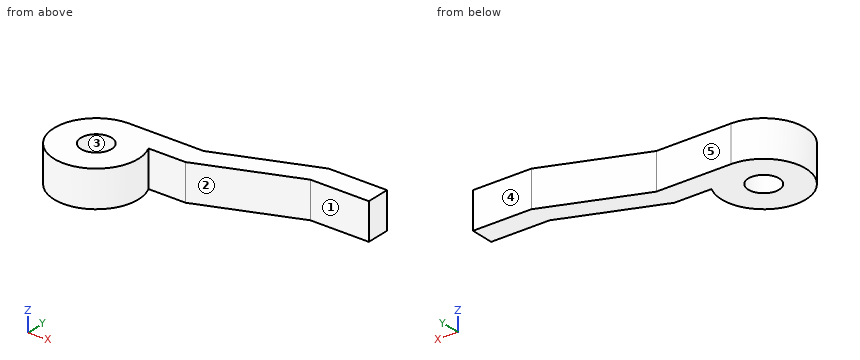
Autodesk Fusion 360 part; units mm, degrees
sketch "Sketch1" plane through (0, 0, 0) normal (0, 0, 1) x (1, 0, 0)
  circle A0 centre (0, 0) radius 0.8344
  line L0 (0, 0) -> (-2.286, 0) construction
  line L1 (0, 2.286) -> (4.064, 2.286)
  line L2 (2.0478, 1.016) -> (4.064, 1.016)
  line L3 (12.446, 4.318) -> (9.271, 4.318)
  line L4 (12.446, 4.318) -> (12.446, 3.048)
  line L5 (12.446, 3.048) -> (9.271, 3.048)
  line L6 (4.064, 2.286) -> (9.271, 4.318)
  line L7 (4.064, 1.016) -> (9.271, 3.048)
  arc A1 (0, 2.286) -> (2.0478, 1.016) centre (0, 0) ccw
  dimension "d1" = 1.6688
  dimension "d2" = 4.572
  dimension "d9" = 3.175
  dimension "d10" = 1.27
  dimension "d11" = 3.175
extrude "Extrude1" add sketch "Sketch1" along normal blind 1.9812
The model under review builds one solid part; all positions refer to its coordinate system, in mm. Face numbers are marked on the shaded views. A direction names the side the tool comes from. Round coordinates to 2 decimals unless told otherwise and drop trailing zeros. Loops run counter-clockwise (first coordinate to the right, second up) from the corner with the lowest first, then second, coordinate; pieces in that order, holes last. Notation, with made-up numbers: M -14.75,-28 L 42.25,-28 A7 ccw 42.25,-16 Z; hole C 40.25,-12 d8. An arc over 180 degrees is marked long. Write item = value, one per line.
Item 1: The part is to be moulded in two halves that separate along X. For the marked faces 1, 2 and 3, say which applies: released by +X, released by -X, zero draft, split by the parting line, or undercut.
Return value:
face_1 = zero draft
face_2 = released by +X
face_3 = undercut
Item 2: For line 1 (Y direction, x = 0, z = 0.75); line 2 (X direction, y = -0.25, z = 1.85); line 3 (Y direction, x = 10.25, z = 1.35), list the stretches that pass through material, from the lowest coordinate up. Write a range as [from, to].
Return value:
line_1 = [-2.29, -0.83], [0.83, 2.29]
line_2 = [-2.27, -0.8], [0.8, 2.27]
line_3 = [3.05, 4.32]
Item 3: Machinability: for the marked faces 4 and 5, which of the approach directions +Z, -Z, +X, -X, +Y, -Y give a long, thin tool a straight path to every point of the face, cutting with its end or side? Answer none if there is none.
Return value:
face_4 = +Z, -Z, +X, -X, +Y
face_5 = +Z, -Z, -X, +Y
Item 4: Take a section at C-C on x = 11.25. Write out the cut boundary in (y, z).
Return value:
outline = M 3.05,0 L 4.32,0 L 4.32,1.98 L 3.05,1.98 Z
Item 5: Take a section at B-B on z = 1.55. Write out the cut boundary in (x, y).
Return value:
outline = M 0,2.29 A2.29 ccw long 2.05,1.02 L 4.06,1.02 L 9.27,3.05 L 12.45,3.05 L 12.45,4.32 L 9.27,4.32 L 4.06,2.29 Z; hole C 0,0 d1.67
Item 6: Take a section at A-A on y = 0. Write out the cut boundary in (x, z), then the cut area to 3 significant figures.
Return value:
outline = M -2.29,0 L -0.83,0 L -0.83,1.98 L -2.29,1.98 Z; M 0.83,0 L 2.29,0 L 2.29,1.98 L 0.83,1.98 Z
area = 5.75 mm2
Item 7: Take a section at D-D on y = -1.5. Write out the cut boundary in (x, z), then the cut area to 3 significant figures.
Return value:
outline = M -1.73,0 L 1.73,0 L 1.73,1.98 L -1.73,1.98 Z
area = 6.84 mm2
Item 8: Insertion check: P1, Ø2, axis at x = 0, y = 0, coming from the +Z side; P2, Ø1, axis at x = 4.5, y = -1, coming from the +Z side (3 decimals); P3, Ø1, axis at x = 3.5, z = 0.5, coming from the -Y side. Each pin has a flat end and moves straight along its axis. Give the tip position at first contact, or say it passes through.
Return value:
P1 = 1.98
P2 = through
P3 = 1.02
